Could you check a few things on this model? Use its own coordinates, in mm. Give positions to 0.01 mm unless a question says otherwise; leave off trailing zeros. Write each loop counter-clockwise with the first axis right and the second up, starting at its lowest first coordinate (ties: lowest second). Pieces come first, ordered by that corner, then holes. Notation, with made-up numbers: (-28, 26.25) - (24, 26.25) arc R20 ccw to (24, 52.25) - close; hole circle Ø4 at (54, 7.25). An arc over 180 degrees is marked (long way). Answer in a Markdown table with one row per item.
from build123d import *

# Parameters (mm, degrees)
F3_SIZE  = 1
F4_SIZE  = 1
F6_R     = 4
F7_DEPTH = 40


with BuildPart() as f2:
    # F0 (on Front) → F2 (revolve)
    with BuildSketch(Plane.XZ):
        Polygon((0, 2), (0, 0), (20, 0), (20, 300), (0, 300), (0, 298), (18, 298), (18, 2), align=None)
    revolve(axis=Axis((0, 0, 152.335405), (0, 0, 1)))

    # F3
    f3_edges = [f2.edges().sort_by_distance(p)[0] for p in [
        (-20, 0, 300),
    ]]
    chamfer(f3_edges, length=F3_SIZE)

    # F4
    f4_edges = [f2.edges().sort_by_distance(p)[0] for p in [
        (-20, 0, 0),
    ]]
    chamfer(f4_edges, length=F4_SIZE)

    # F6 (on offset) → F7 (cut)
    with BuildSketch(Plane.XZ.offset(20)):
        with Locations((0, 25)):
            Circle(F6_R)
    extrude(amount=-F7_DEPTH, mode=Mode.SUBTRACT)


solid = f2.part
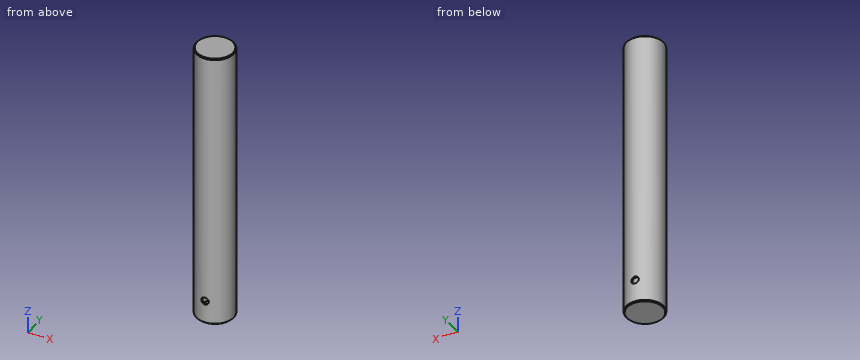
1) Imagine slicing it at C-C (z = 85.5). List the corners of the cut face in (x, y) for me, then the cut area to 3 significant figures.
Check values:
| item | result |
|---|---|
| outline | circle Ø40 at (0, 0); hole circle Ø36 at (0, 0) |
| area | 239 mm2 |
2) Will these pins go through, and if not, where does the flat tip stop? P1, Ø2, axis at x = 13.5, z = 228.5, coming from the +Y side; P2, Ø1, axis at x = 11.5, z = 117, coming from the -Y side; P3, Ø1.5, axis at y = -1, z = 226.5, coming from the +X side.
Check values:
| item | result |
|---|---|
| P1 | stops at y = 15.61 |
| P2 | stops at y = -16.7 |
| P3 | stops at x = 20 |
3) Imagine slicing it at A-A (x = 0). List the corners of the cut face in (y, z) for me, then the cut area to 3 significant figures.
Check values:
| item | result |
|---|---|
| outline | (-20, 1) - (-19, 0) - (19, 0) - (20, 1) - (20, 21) - (18, 21) - (18, 2) - (-18, 2) - (-18, 21) - (-20, 21) - close; (-20, 29) - (-18, 29) - (-18, 298) - (18, 298) - (18, 29) - (20, 29) - (20, 299) - (19, 300) - (-19, 300) - (-20, 299) - close |
| area | 1,310 mm2 |
4) If I drill on line 1 (Z direction, x = -0.5, y = -6); line 2 (X direction, y = 0.5, z = 264.5); line 3 (Y direction, x = 0, z = 186), over which ranges is the centre line in solid material (lowest first)?
Check values:
| item | result |
|---|---|
| line 1 | z = 0 to 2, 298 to 300 |
| line 2 | x = -19.99 to -17.99, 17.99 to 19.99 |
| line 3 | y = -20 to -18, 18 to 20 |
5) Imagine slicing it at B-B (z = 25). List the corners of the cut face in (x, y) for me, then the cut area to 3 significant figures.
Check values:
| item | result |
|---|---|
| outline | (-4, -19.6) - (-4, -17.55) arc R18 cw to (-4, 17.55) - (-4, 19.6) arc R20 ccw to start; (4, -19.6) arc R20 ccw to (4, 19.6) - (4, 17.55) arc R18 cw to (4, -17.55) - close |
| area | 207 mm2 |
